```python
from build123d import *

# Parameters (mm, degrees)
SKETCH_1_W          = 40
SKETCH_1_H          = 8
SKETCH_1_R          = 1.5
EXTRUDE_1_DEPTH     = 10
SKETCH_2_R          = 1.5
CUT_EXTRUDE_5_DEPTH = 9


with BuildPart() as part:
    # 草图1 → 凸台-拉伸1 (new body)
    with BuildSketch(Plane.XY):
        Rectangle(SKETCH_1_W, SKETCH_1_H)
        with Locations((-15, 0)):
            Circle(SKETCH_1_R, mode=Mode.SUBTRACT)
        with Locations((5, 0)):
            Circle(SKETCH_1_R, mode=Mode.SUBTRACT)
    extrude(amount=EXTRUDE_1_DEPTH)

    # 草图2 → 切除-拉伸5 (cut, through all)
    with BuildSketch(Plane(origin=(0, 4, 0), x_dir=(1, 0, 0), z_dir=(0, 1, 0))):
        with Locations((15, -5)):
            Circle(SKETCH_2_R)
        with Locations((-5, -5)):
            Circle(SKETCH_2_R)
    extrude(amount=-CUT_EXTRUDE_5_DEPTH, mode=Mode.SUBTRACT)


solid = part.part
```
Geometry check sheet. Reference: the model listing, model coordinates, mm. Round coordinates to 2 decimals unless told otherwise and drop trailing zeros. Loops run counter-clockwise (first coordinate to the right, second up) from the corner with the lowest first, then second, coordinate; pieces in that order, holes last. Notation, with made-up numbers: (-4.75, 8) - (20.25, 8) arc R33 ccw to (20.25, 45) - close; hole circle Ø9 at (-25, -16). An arc over 180 degrees is marked (long way). Write each question's results on one line, items separated by ' | '. Start each with the question number.
Q1. Cross-section at A-A on y = 0. Enter the section's corners in (x, z).
Q2. Cross-section at D-D on y = -2.25. Enter the section's corners in (x, z).
Q3. Cross-section at C-C on x = -15. Enter the section's corners in (y, z).
Q4. Gauge pin test, flat ends, axial feed: P1, Ø3.5, axis at x = 15, z = 5, coming from the +Y side; P2, Ø1.8, axis at x = -15, y = 0, coming from the +Z side. Record the tip position at first contact, or that the pin passes through.
Q5. Cross-section at B-B on z = 5. Enter the section's corners in (x, y), and give its area (3 significant figures).
Q6. Release check for a two-part mould opening along Y. For faces 1 (the flat face through (0, 4, 5)), 2 (the cylindrical face through (6.386, -0.575, 4.93)), 3 (the flat face through (0, 0, 10)) record: +Y half, -Y half, draft (parallel to the pull), parting line (faces both ways), or undercut.
Q7. Thickness scan on line 1 (Z direction, x = -5, y = -1.5); line 2 (Y direction, x = 5, z = 1.25); line 3 (X direction, y = -3.5, z = 4.75). Record the ranges inside material, lowest first. Write a range as [from, to].
Answers below:
1) outline: (-20, 0) - (-16.5, 0) - (-16.5, 10) - (-20, 10) - close; (-13.5, 0) - (3.5, 0) - (3.5, 10) - (-13.5, 10) - close; (6.5, 0) - (20, 0) - (20, 10) - (6.5, 10) - close; hole circle Ø3 at (-5, 5); hole circle Ø3 at (15, 5)
2) outline: (-20, 0) - (20, 0) - (20, 10) - (-20, 10) - close; hole circle Ø3 at (-5, 5); hole circle Ø3 at (15, 5)
3) outline: (-4, 0) - (-1.5, 0) - (-1.5, 10) - (-4, 10) - close; (1.5, 0) - (4, 0) - (4, 10) - (1.5, 10) - close
4) P1: stops at y = 4 | P2: passes through
5) outline: (-20, -4) - (-6.5, -4) - (-6.5, 4) - (-20, 4) - close; (-3.5, -4) - (13.5, -4) - (13.5, 4) - (-3.5, 4) - close; (16.5, -4) - (20, -4) - (20, 4) - (16.5, 4) - close; hole circle Ø3 at (-15, 0); hole circle Ø3 at (5, 0) | area: 258 mm²
6) face 1: +Y half | face 2: undercut | face 3: draft
7) line 1: z = [0, 3.5], [6.5, 10] | line 2: y = [-4, -1.5], [1.5, 4] | line 3: x = [-20, -6.48], [-3.52, 13.52], [16.48, 20]
